The model under review builds one solid part; all positions refer to its coordinate system, in mm. Face numbers are marked on the shaded views. A direction names the side the tool comes from. Round coordinates to 2 decimals unless told otherwise and drop trailing zeros. Write each loop counter-clockwise with the first axis right and the second up, starting at its lowest first coordinate (ties: lowest second). Pieces come first, ordered by that corner, then holes. Notation, with made-up numbers: (-12.75, 37.25) - (21.25, 37.25) arc R25 ccw to (21.25, 66.25) - close; hole circle Ø3 at (55, 42.5). An arc over 180 degrees is marked (long way). Return JSON: item names as keys, results as strings.
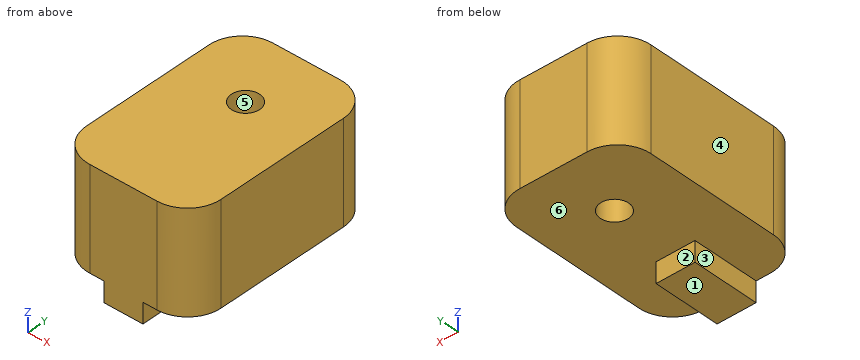
from build123d import *

# Parameters (mm, degrees)
SKETCH_2_W      = 20
SKETCH_2_H      = 30
SKETCH_2_R      = 2.1
EXTRUDE_1_DEPTH = 15
SKETCH_3_W      = 5.8
SKETCH_3_H      = 10
EXTRUDE_2_DEPTH = 3
FILLET_1_R      = 5


with BuildPart() as part:
    # ｽｹｯﾁ2 → ﾎﾞｽ - 押し出し1 (new body)
    with BuildSketch(Plane.XY):
        Rectangle(SKETCH_2_W, SKETCH_2_H)
        with Locations((0, 5)):
            Circle(SKETCH_2_R, mode=Mode.SUBTRACT)
    extrude(amount=EXTRUDE_1_DEPTH)

    # ｽｹｯﾁ3 → ﾎﾞｽ - 押し出し2 (add)
    with BuildSketch(Plane(origin=(0, 0, 0), x_dir=(-1, 0, 0), z_dir=(0, 0, -1))):
        with Locations((0, -10)):
            Rectangle(SKETCH_3_W, SKETCH_3_H)
    extrude(amount=EXTRUDE_2_DEPTH)

    # ﾌｨﾚｯﾄ1
    fillet_1_edges = [part.edges().sort_by_distance(p)[0] for p in [
        (10, -15, 7.5),
        (-10, -15, 7.5),
        (-10, 15, 7.5),
        (10, 15, 7.5),
    ]]
    fillet(fillet_1_edges, radius=FILLET_1_R)


solid = part.part
(1) Add section D-D (y = 5). Write out the cut boundary in (x, z).
Filled in:
{"outline": "(-10, 0) - (-2.1, 0) - (-2.1, 15) - (-10, 15) - close; (2.1, 0) - (10, 0) - (10, 15) - (2.1, 15) - close"}
(2) For the marked faces 1, 2 and 3, list the 3-axis set-ups (+Z, -Z, +X, -X, +Y, -Y) from which the entire face can be reached by the end or side of a thin tool; tool diameter is ignored.
Filled in:
{"face 1": "-Z, +X, -X, +Y, -Y", "face 2": "-Z, +X, -X, +Y", "face 3": "-Z, -X, +Y, -Y"}
(3) Mouldability with a two-part tool opening along X and no side actions: class the marked faces 4, 5 and 6 as released by +X, released by -X, zero draft, split by the parting line, or undercut.
Filled in:
{"face 4": "released by -X", "face 5": "undercut", "face 6": "zero draft"}
(4) Add section C-C (z = 13.5). Write out the cut boundary in (x, y), plus the area to 3 significant figures.
Filled in:
{"outline": "(-10, -10) arc R5 ccw to (-5, -15) - (5, -15) arc R5 ccw to (10, -10) - (10, 10) arc R5 ccw to (5, 15) - (-5, 15) arc R5 ccw to (-10, 10) - close; hole circle Ø4.2 at (0, 5)", "area": "565 mm2"}
(5) Wall thickness on line 1 (Z direction, x = 4.75, y = -3.75); line 2 (Y direction, x = 0, z = 11.25); line 3 (Y direction, x = 1.5, z = 6): over which ranges is each line inside the solid? List them lowest first.
Filled in:
{"line 1": "z = 0 to 15", "line 2": "y = -15 to 2.9, 7.1 to 15", "line 3": "y = -15 to 3.53, 6.47 to 15"}
(6) Clearance check with flat-ended pins moving along their axes: pin 1 Ø8 at (x, z) = (7.5, 8.5) entering from -Y; pin 2 Ø1.5 at (y, z) = (11.5, 2.5) entering from -X; pin 3 Ø2.5 at (y, z) = (-8.5, -1.5) entering from -X; pin 4 Ø0.9 at (y, z) = (-11.5, -2) entering from +X. State where each tip first meets the part, or that it passes through.
Filled in:
{"pin 1": "stops at y = -15", "pin 2": "stops at x = -9.94", "pin 3": "stops at x = -2.9", "pin 4": "stops at x = 2.9"}
(7) Add section A-A (x = 0). Write out the cut boundary in (y, z).
Filled in:
{"outline": "(-15, -3) - (-5, -3) - (-5, 0) - (2.9, 0) - (2.9, 15) - (-15, 15) - close; (7.1, 0) - (15, 0) - (15, 15) - (7.1, 15) - close"}
(8) Add section B-B (y = -8.5). Write out the cut boundary in (x, z).
Filled in:
{"outline": "(-10, 0) - (-2.9, 0) - (-2.9, -3) - (2.9, -3) - (2.9, 0) - (10, 0) - (10, 15) - (-10, 15) - close"}
